```python
from build123d import *

# Parameters (mm, degrees)
BOSS_EXTRUDE1_DEPTH = 12.7
SKETCH2_W           = 40
SKETCH2_H           = 12.7
SKETCH2_W_2         = 60
SKETCH2_H_2         = 40
CUT_EXTRUDE1_DEPTH  = 12.7


with BuildPart() as part:
    # Sketch1 → Boss-Extrude1 (new body)
    with BuildSketch(Plane(origin=(0, 0, 0), x_dir=(1, 0, 0), z_dir=(0, 1, 0))):
        Polygon((-127.7, -137.3), (-20, -137.3), (-20, -150), (20, -150), (20, -137.3), (127.7, -137.3), (127.7, -20), (140.4, -20), (140.4, 20), (127.7, 20), (127.7, 137.3), (20, 137.3), (20, 150), (-20, 150), (-20, 137.3), (-127.7, 137.3), (-127.7, 20), (-140.4, 20), (-140.4, -20), (-127.7, -20), align=None)
    extrude(amount=BOSS_EXTRUDE1_DEPTH)

    # Sketch2 → Cut-Extrude1 (cut)
    with BuildSketch(Plane(origin=(0, 12.7, 0), x_dir=(1, 0, 0), z_dir=(0, 1, 0))):
        with Locations((-75.7, 13.65)):
            Rectangle(SKETCH2_W, SKETCH2_H)
        with Locations((75.7, 13.65)):
            Rectangle(SKETCH2_W, SKETCH2_H)
        with Locations((0, 60)):
            Rectangle(SKETCH2_W_2, SKETCH2_H_2)
    extrude(amount=-CUT_EXTRUDE1_DEPTH, mode=Mode.SUBTRACT)


solid = part.part
```
Could you check a few things on this model? Use its own coordinates, in mm. A direction names the side the tool comes from. Coordinates: 2 decimals unless noted, no trailing zeros. Order: outer loops, then holes, each group sorted by start corner. A loop starts at its lowest first (then second) coordinate and runs counter-clockwise, first axis right, second up. Notation, with made-up numbers: M 80.5,7 L 90.5,7 A20 ccw 90.5,45 Z; hole C 15.25,6.5 d2. An arc over 180 degrees is marked long. Use a Markdown table: item, result. Add a question column.
Q1. I'm going to push flat-ended pins straight in: pin 1 (3 mm diameter, centred on y = 3.5, z = -51.5, fed in from +X); pin 2 (4 mm diameter, centred on x = -134.5, y = 4.5, fed in from -Z); pin 3 (1 mm diameter, centred on y = 4.5, z = 91, fed in from -X). Where does each tip first touch, or does it pass through?
Q2. We'd pull the mould along X, two halves only. Please class faces 4 (the flat face through (-55.7, 6, -14)), 5 (the flat face through (20, 6, 144)), 6 (the flat face through (0, 6, -150)): pulls with the +X half, pulls with the -X half, needs draft (parallel to the pull), parting line crosses it, or undercut.
Q3. I want a section at D-D on z = 80. List the corners of the cut face in (x, y) for me, then the cut area to 3 significant figures.
Q4. I want a section at C-C on z = -64. List the corners of the cut face in (x, y) for me, then the cut area to 3 significant figures.
Q5. If I drill on L1, parallel to X at y = 10.25, z = -71; L2, parallel to Z at x = -91.5, y = 12; L3, parallel to X at y = 2.5, z = -98.5, over which ranges is the centre line in solid material (lowest first)?
Q6. I want a section at A-A on x = 81.5. List the corners of the cut face in (y, z) for me.
Q7. Which directions (+Z, -Z, +X, -X, +Y, -Y) give clear straight access to the entire face, cutting with the end or side of a thin tool? Please do faces 1 (the flat face through (-20, 6, -144)), 2 (the flat face through (-75, 6, 137.3)), 3 (the flat face through (95.7, 6, -14)).
Q8. I want a section at B-B on y = 2.5. Give the number of separate pieces and of enclosed holes in the cut face, then the cut area to 3 significant figures.
Checked values:
| question | item | result |
|---|---|---|
| 1 | pin 1 | x = 127.7 |
| 1 | pin 2 | z = -20 |
| 1 | pin 3 | x = -127.7 |
| 2 | face 4 | undercut |
| 2 | face 5 | pulls with the +X half |
| 2 | face 6 | needs draft |
| 3 | outline | M -127.7,0 L 127.7,0 L 127.7,12.7 L -127.7,12.7 Z |
| 3 | area | 3,240 mm² |
| 4 | outline | M -127.7,0 L -30,0 L -30,12.7 L -127.7,12.7 Z; M 30,0 L 127.7,0 L 127.7,12.7 L 30,12.7 Z |
| 4 | area | 2,480 mm² |
| 5 | L1 | -127.7 to -30, 30 to 127.7 |
| 5 | L2 | -137.3 to -20, -7.3 to 137.3 |
| 5 | L3 | -127.7 to 127.7 |
| 6 | outline | M 0,-137.3 L 12.7,-137.3 L 12.7,-20 L 0,-20 Z; M 0,-7.3 L 12.7,-7.3 L 12.7,137.3 L 0,137.3 Z |
| 7 | face 1 | -Z, -X, +Y, -Y |
| 7 | face 2 | +Z, -X, +Y, -Y |
| 7 | face 3 | +Y, -Y |
| 8 | separate pieces | 1 |
| 8 | enclosed holes | 3 |
| 8 | area | 68,700 mm² |
